Verification items for this drawing (mm, ordinates from the low corner). A direction names the side the tool comes from. Give positions to 0.01 mm unless a question says otherwise; leave off trailing zeros. Write each loop counter-clockwise with the first axis right and the second up, starting at its lowest first coordinate (ties: lowest second). Pieces come first, ordered by that corner, then holes. Notation, with made-up numbers: (46, 69.25) -> (56, 69.25) arc R37 ccw to (56, 107.25) -> close; hole circle Ø7 at (-37.75, 30.25). An arc over 180 degrees is marked (long way). Write item = value, one per line.
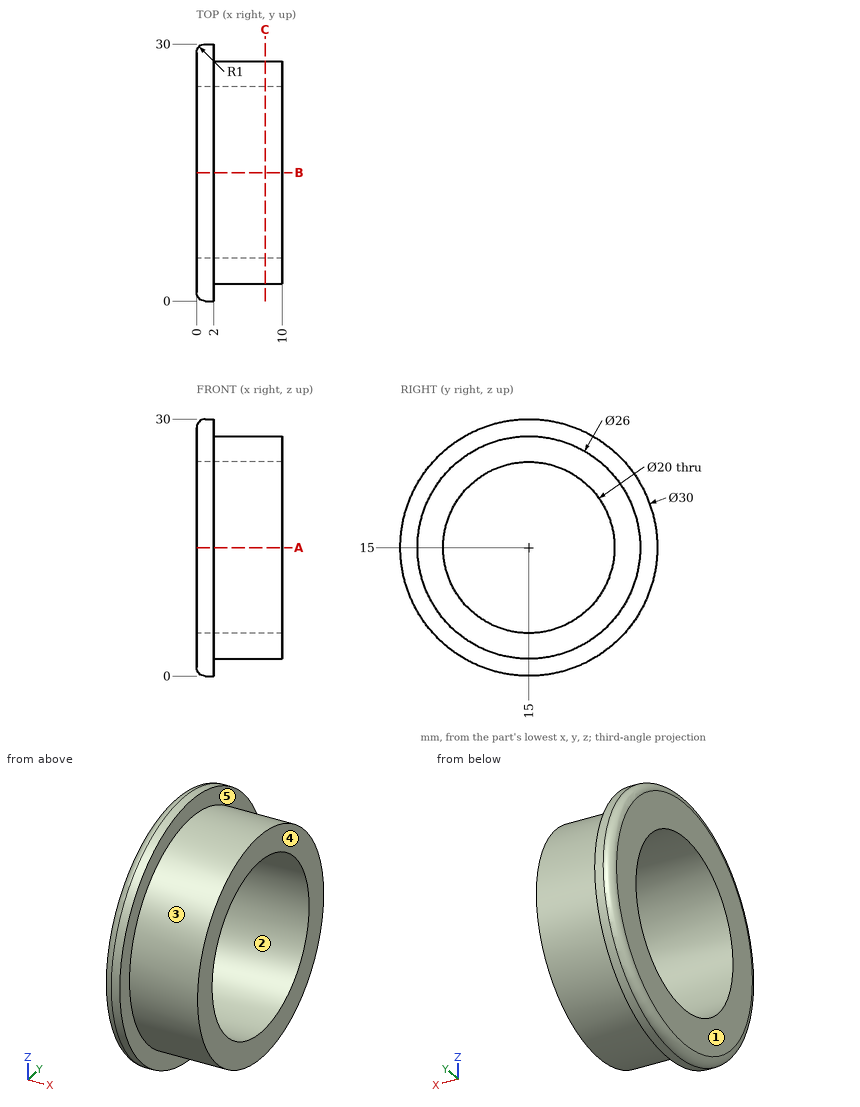
Item 1: Sectioned sample at C-C on x = 8. Record the cut outline in (y, z), then the cut area to 3 significant figures.
Response values:
outline = circle Ø26 at (15, 15); hole circle Ø20 at (15, 15)
area = 217 mm^2
Item 2: Go/stop test with flat-tipped pins: P1, Ø6, axis at x = 5.5, z = 4, coming from the -Y side; P2, Ø18, axis at y = 15, z = 15, coming from the +X side; P3, Ø12, axis at y = 3.5, z = 14.5, coming from the -X side; P4, Ø6, axis at x = 7, z = 14, coming from the +Y side. Record where each tip stops, or that it passes through.
Response values:
P1 = 4.75
P2 = through
P3 = 0
P4 = 28
Item 3: Set-up check for the marked faces 4 and 5: record each of +Z, -Z, +X, -X, +Y, -Y from which the full face is reachable in a straight line by a thin tool's end or side.
Response values:
face_4 = +Z, -Z, +X, +Y, -Y
face_5 = +X
Item 4: Material ranges on line 1 (Z direction, x = 6.5, y = 15); line 2 (Y direction, x = 4, z = 9.5), recorded low to high.
Response values:
line_1 = 2 to 5, 25 to 28
line_2 = 3.22 to 6.65, 23.35 to 26.78
Item 5: Mould release check, pull along Y, two halves, no side actions. Record for the marked faces 1, 2 and 3: +Y half, -Y half, draft (parallel to the pull), parting line (faces both ways), or undercut.
Response values:
face_1 = draft
face_2 = undercut
face_3 = parting line
Item 6: Sectioned sample at A-A on z = 15. Record the cut outline in (x, y), then the cut area to 3 significant figures.
Response values:
outline = (0, 1) arc R1 ccw to (1, 0) -> (2, 0) -> (2, 2) -> (10, 2) -> (10, 5) -> (0, 5) -> close; (0, 25) -> (10, 25) -> (10, 28) -> (2, 28) -> (2, 30) -> (1, 30) arc R1 ccw to (0, 29) -> close
area = 67.6 mm^2
